Check sheet for the drawn part. Datum: minimum x, y, z corner. Units: mm. A direction names the side the tool comes from. Give positions to 0.01 mm unless a question says otherwise; leave off trailing zeros. Loops run counter-clockwise (first coordinate to the right, second up) from the corner with the lowest first, then second, coordinate; pieces in that order, holes last.
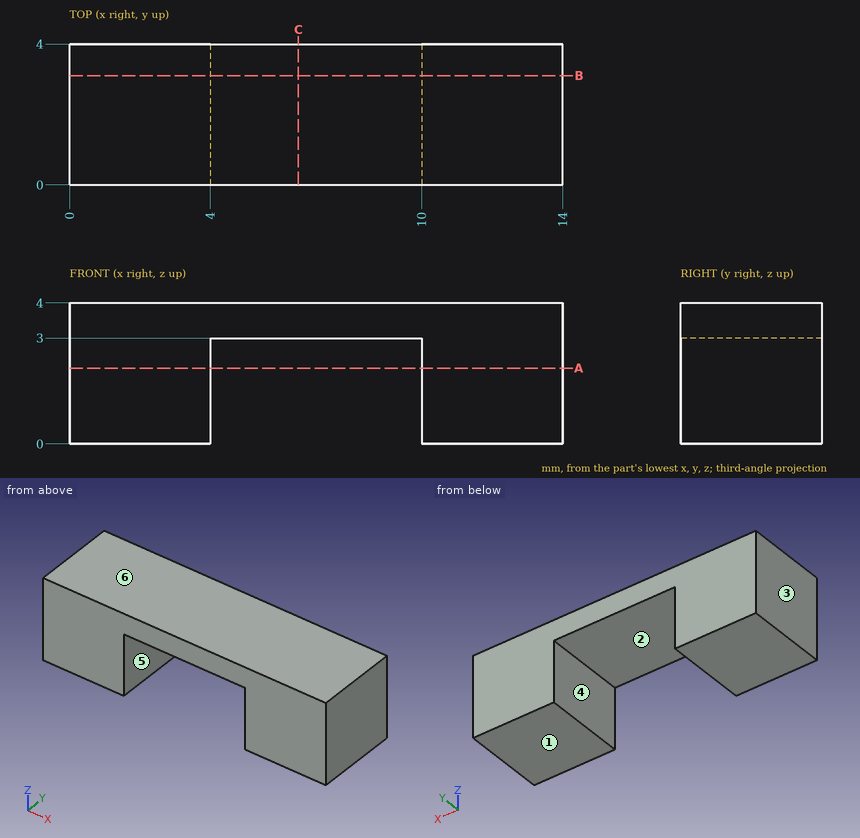
(1) Section check A-A on z = 2.15. Record the boundary of the cut face in (x, y), plus the area to 3 significant figures.
(2) Section check C-C on x = 6.5. Record the boundary of the cut face in (y, z), plus the area to 3 significant figures.
(3) Release check for a two-part mould opening along X. For the marked faces 3, 4, 5 and 6 record: pulls with the +X half, pulls with the -X half, needs draft (parallel to the pull), parting line crosses it, or undercut.
(4) Access from +Z, -Z, +X, -X, +Y, -Y to the whole of each face (thin tool, end or side, straight path). Record for the marked faces 1 and 2.
(5) Material ranges on line 1 (X direction, y = 2.3, z = 0.3); line 2 (Z direction, x = 8.25, y = 0.9), recorded low to high.
(6) Section check B-B on y = 3.1. Record the boundary of the cut face in (x, z).
Computed values:
1. outline: (0, 0) - (4, 0) - (4, 4) - (0, 4) - close; (10, 0) - (14, 0) - (14, 4) - (10, 4) - close
1. area: 32.0 mm2
2. outline: (0, 3) - (4, 3) - (4, 4) - (0, 4) - close
2. area: 4.00 mm2
3. face 3: pulls with the -X half
3. face 4: undercut
3. face 5: undercut
3. face 6: needs draft
4. face 1: -Z, +X, -X, +Y, -Y
4. face 2: -Z, +Y, -Y
5. line 1: x = 0 to 4, 10 to 14
5. line 2: z = 3 to 4
6. outline: (0, 0) - (4, 0) - (4, 3) - (10, 3) - (10, 0) - (14, 0) - (14, 4) - (0, 4) - close
